```python
from build123d import *

# Parameters (mm, degrees)
F0_W     = 60
F0_H     = 60
F1_DEPTH = 45
F2_T     = -2
F3_W     = 2.8
F3_H     = 7
F4_DEPTH = 64.2
F5_W     = 2.8
F5_H     = 7
F6_DEPTH = 63.5
F8_DEPTH = 25
F9_R     = 3
F10_R    = 1


# Not quite as in the source:
# - a feature names something its author has since deleted; it is built from what else it names


with BuildPart() as f1:
    # F0 (on Top) → F1 (new body)
    with BuildSketch(Plane.XY):
        Rectangle(F0_W, F0_H)
    extrude(amount=F1_DEPTH)

    # F2
    f2_openings = [f1.faces().sort_by_distance(p)[0] for p in [
        (0, 0, 45),
    ]]
    offset(amount=F2_T, openings=f2_openings)

    # F3 (on face) → F4 (cut)
    with BuildSketch(Plane.XZ.offset(30)):
        Polygon((-15.0992558567, 35), (-6, 10), (-4, 10), (-4, 17), (-11.0992558567, 35), align=None)
        with Locations((-1.8, 13.5)):
            Rectangle(F3_W, F3_H)
        with Locations((1.8, 13.5)):
            Rectangle(F3_W, F3_H)
        Polygon((4, 17), (4, 10), (6, 10), (15.0992558567, 35), (11.0992558567, 35), align=None)
    extrude(amount=-F4_DEPTH, mode=Mode.SUBTRACT)

    # F5 (on face) → F6 (cut)
    with BuildSketch(Plane.YZ.offset(30)):
        Polygon((-15.0992558567, 35), (-6, 10), (-4, 10), (-4, 17), (-11.0992558567, 35), align=None)
        with Locations((-1.8, 13.5)):
            Rectangle(F5_W, F5_H)
        with Locations((1.8, 13.5)):
            Rectangle(F5_W, F5_H)
        Polygon((4, 17), (4, 10), (6, 10), (15.0992558567, 35), (11.0992558567, 35), align=None)
    extrude(amount=-F6_DEPTH, mode=Mode.SUBTRACT)

    # F7 (on face) → F8 (cut)
    with BuildSketch(Plane(origin=(0, 0, 0), x_dir=(1, 0, 0), z_dir=(0, 0, -1))):
        with BuildLine():
            Line((0.9656854249, 0.4), (9.9919967974, 0.4))
            ThreePointArc((9.9919967974, 0.4), (9.2387953251, 3.8268343237), (7.3482514055, 6.7825659806))
            Line((7.3482514055, 6.7825659806), (0.9656854249, 0.4))
        make_face()
        with BuildLine():
            ThreePointArc((7.3482514055, -6.7825659806), (9.2387953251, -3.8268343237), (9.9919967974, -0.4))
            Line((9.9919967974, -0.4), (0.9656854249, -0.4))
            Line((0.9656854249, -0.4), (7.3482514055, -6.7825659806))
        make_face()
        with BuildLine():
            Line((0.4, 0.9656854249), (6.7825659806, 7.3482514055))
            ThreePointArc((6.7825659806, 7.3482514055), (3.8268343237, 9.2387953251), (0.4, 9.9919967974))
            Line((0.4, 9.9919967974), (0.4, 0.9656854249))
        make_face()
        with BuildLine():
            ThreePointArc((0.4, -9.9919967974), (3.8268343237, -9.2387953251), (6.7825659806, -7.3482514055))
            Line((6.7825659806, -7.3482514055), (0.4, -0.9656854249))
            Line((0.4, -0.9656854249), (0.4, -9.9919967974))
        make_face()
        with BuildLine():
            Line((-6.7825659806, 7.3482514055), (-0.4, 0.9656854249))
            Line((-0.4, 0.9656854249), (-0.4, 9.9919967974))
            ThreePointArc((-0.4, 9.9919967974), (-3.8268343237, 9.2387953251), (-6.7825659806, 7.3482514055))
        make_face()
        with BuildLine():
            Line((-0.4, -9.9919967974), (-0.4, -0.9656854249))
            Line((-0.4, -0.9656854249), (-6.7825659806, -7.3482514055))
            ThreePointArc((-6.7825659806, -7.3482514055), (-3.8268343237, -9.2387953251), (-0.4, -9.9919967974))
        make_face()
        with BuildLine():
            Line((-7.3482514055, -6.7825659806), (-0.9656854249, -0.4))
            Line((-0.9656854249, -0.4), (-9.9919967974, -0.4))
            ThreePointArc((-9.9919967974, -0.4), (-9.2387953251, -3.8268343237), (-7.3482514055, -6.7825659806))
        make_face()
        with BuildLine():
            Line((-9.9919967974, 0.4), (-0.9656854249, 0.4))
            Line((-0.9656854249, 0.4), (-7.3482514055, 6.7825659806))
            ThreePointArc((-7.3482514055, 6.7825659806), (-9.2387953251, 3.8268343237), (-9.9919967974, 0.4))
        make_face()
    extrude(amount=-F8_DEPTH, mode=Mode.SUBTRACT)

    # F9
    f9_edges = [f1.edges().sort_by_distance(p)[0] for p in [
        (-30, -30, 22.5),
        (30, -30, 22.5),
        (30, 30, 22.5),
        (-30, 30, 22.5),
        (-28, -28, 23.5),
        (28, -28, 23.5),
        (28, 28, 23.5),
        (-28, 28, 23.5),
    ]]
    fillet(f9_edges, radius=F9_R)

    # F10
    f10_edges = [f1.edges().sort_by_distance(p)[0] for p in [
        (0, -30, 0),
        (-30, 0, 0),
        (30, 0, 0),
        (0, 30, 0),
        (29.12132, 29.12132, 0),
        (-29.12132, 29.12132, 0),
        (29.12132, -29.12132, 0),
        (-29.12132, -29.12132, 0),
    ]]
    fillet(f10_edges, radius=F10_R)


solid = f1.part
```
Geometry check sheet. Reference: the model listing, model coordinates, mm. A direction names the side the tool comes from. Give positions to 0.01 mm unless a question says otherwise; leave off trailing zeros. Write each loop counter-clockwise with the first axis right and the second up, starting at its lowest first coordinate (ties: lowest second). Pieces come first, ordered by that corner, then holes.
1) Gauge pin test, flat ends, axial feed: pin 1 (1 mm diameter, centred on x = 28.5, z = 14, fed in from -Y); pin 2 (2 mm diameter, centred on x = -29.5, z = 12.5, fed in from -Y); pin 3 (12 mm diameter, centred on x = 14.5, z = 33.5, fed in from +Y); pin 4 (17 mm diameter, centred on x = -0.5, y = -11, fed in from +Z). Record the tip position at first contact, or that the pin passes through.
2) Material ranges on L1, parallel to Y at x = 18.5, z = 29; L2, parallel to Z at x = -11, y = -4.5, recorded low to high.
3) Section check B-B, the plane y = 22.5. Record the boundary of the cut face in (x, z), and give its area (3 significant figures).
4) Release check for a two-part mould opening along X. For faces 1 (the cylindrical face through (-29.14, -29.1, 23.31)), 2 (the flat face through (-28.99, -7.5, 25.87)), 3 (the flat face through (-3.636, -4.202, 0.986)) record: pulls with the +X half, pulls with the -X half, needs draft (parallel to the pull), parting line crosses it, or undercut.
5) Section check A-A, the plane z = 37. Record the boundary of the cut face in (x, y), and give its area (3 significant figures).
6) Section check D-D, the plane y = -9. Record the boundary of the cut face in (x, z).
7) Section check C-C, the plane x = -13. Record the boundary of the cut face in (y, z), and give its area (4 significant figures).
8) Access from +Z, -Z, +X, -X, +Y, -Y to the whole of each face (thin tool, end or side, straight path). Record for faces 4 (the flat face through (0, 0, 2)), 5 (the flat face through (29, 0.4, 13)), 6 (the flat face through (-10.61, -29.01, 22.67)), 7 (the cylindrical face through (-29.14, 29.1, 23.31)), 8 (the flat face through (-0.4, 6, 1)).
Computed:
1. pin 1: stops at y = -29.83
1. pin 2: stops at y = -29.6
1. pin 3: stops at y = 30
1. pin 4: stops at z = 2
2. L1: y = -30 to -28, 28 to 30
2. L2: z = 0 to 2
3. outline: (-30, 1) arc R1 ccw to (-29, 0) - (29, 0) arc R1 ccw to (30, 1) - (30, 45) - (28, 45) - (28, 2) - (-28, 2) - (-28, 45) - (-30, 45) - close
3. area: 292 mm2
4. face 1: pulls with the -X half
4. face 2: needs draft
4. face 3: undercut
5. outline: (-30, -27) arc R3 ccw to (-27, -30) - (27, -30) arc R3 ccw to (30, -27) - (30, 27) arc R3 ccw to (27, 30) - (-27, 30) arc R3 ccw to (-30, 27) - close; hole (-28, -25) arc R3 ccw to (-25, -28) - (25, -28) arc R3 ccw to (28, -25) - (28, 25) arc R3 ccw to (25, 28) - (-25, 28) arc R3 ccw to (-28, 25) - close
5. area: 464 mm2
6. outline: (-30, 1) arc R1 ccw to (-29, 0) - (-4.36, 0) - (-4.36, 2) - (-28, 2) - (-28, 18.24) - (-30, 18.24) - close; (-30, 29.68) - (-28, 29.68) - (-28, 45) - (-30, 45) - close; (-0.4, 0) - (0.4, 0) - (0.4, 2) - (-0.4, 2) - close; (4.36, 0) - (29, 0) arc R1 ccw to (30, 1) - (30, 18.24) - (28, 18.24) - (28, 2) - (4.36, 2) - close; (28, 29.68) - (30, 29.68) - (30, 45) - (28, 45) - close
7. outline: (-30, 1) arc R1 ccw to (-29, 0) - (29, 0) arc R1 ccw to (30, 1) - (30, 29.23) - (28, 29.23) - (28, 2) - (-28, 2) - (-28, 29.23) - (-30, 29.23) - close; (-30, 35) - (-28, 35) - (-28, 45) - (-30, 45) - close; (28, 35) - (30, 35) - (30, 45) - (28, 45) - close
7. area: 268.5 mm2
8. face 4: +Z
8. face 5: +X, -X
8. face 6: +Y, -Y
8. face 7: +Z, -Z, -X, +Y
8. face 8: +Z, -Z
